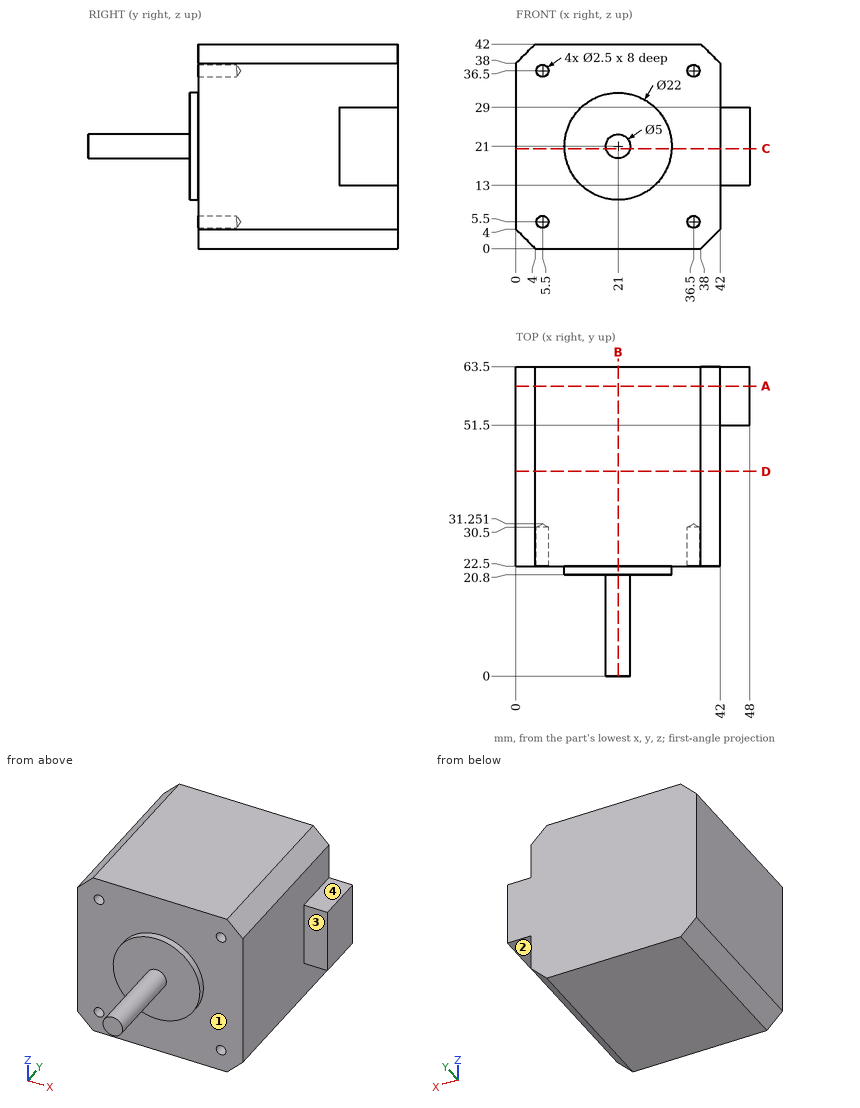
Print and shaded views of the part. All mm, measured from the part's lowest x, y and z. A direction names the side the tool comes from. Coordinates: 2 decimals unless noted, no trailing zeros. Loops run counter-clockwise (first coordinate to the right, second up) from the corner with the lowest first, then second, coordinate; pieces in that order, holes last. Notation, with made-up numbers: (15.25, 44.25) - (35.25, 44.25) arc R23 cw to (35.25, 56.25) - close; hole circle Ø3 at (-5, -13). An arc over 180 degrees is marked (long way). Write item = value, one per line. Start each with the question number.
Item 1: Cut at D-D, the plane y = 42. Give the cut face in (x, z).
Item 2: Cut at B-B, the plane x = 21. Give the cut face in (y, z), and give its area (3 significant figures).
Item 3: 3-axis set-ups, long thin cutter, end or side, ignore diameter. For the marked faces 1, 2, 3 and 4: which of +Z, -Z, +X, -X, +Y, -Y reach the whole face in a straight line?
Item 4: Wall check: L1, parallel to X at y = 25.5, z = 5.5; L2, parallel to X at y = 28, z = 36. Give the ranges that are in metal, low to high. Write a range as from..to.
Item 5: Cut at C-C, the plane z = 20.5. Give the cut face in (x, y).
Item 6: Flat gauge pins, fed straight in: pin 1 Ø5 at (x, y) = (46, 60) entering from +Z; pin 2 Ø1.8 at (x, y) = (45.5, 54.5) entering from -Z; pin 3 Ø1 at (y, z) = (25, 7.5) entering from +X; pin 4 Ø11 at (x, z) = (22.5, 21.5) entering from -Y. Where does each tip first touch, or does it go through?
Item 7: Cut at A-A, the plane y = 59.5. Give the cut face in (x, z).
The answers:
q1.outline = (0, 4) - (4, 0) - (38, 0) - (42, 4) - (42, 38) - (38, 42) - (4, 42) - (0, 38) - close
q2.outline = (0, 18.5) - (20.8, 18.5) - (20.8, 10) - (22.5, 10) - (22.5, 0) - (63.5, 0) - (63.5, 42) - (22.5, 42) - (22.5, 32) - (20.8, 32) - (20.8, 23.5) - (0, 23.5) - close
q2.area = 1,860 mm2
q3.face_1 = -Y
q3.face_2 = -Z, +X, +Y, -Y
q3.face_3 = +Z, -Z, +X, -Y
q3.face_4 = +Z, +X, +Y, -Y
q4.L1 = 0..4.25, 6.75..35.25, 37.75..42
q4.L2 = 0..4.35, 6.65..35.35, 37.65..42
q5.outline = (0, 22.5) - (10.01, 22.5) - (10.01, 20.8) - (18.55, 20.8) - (18.55, 0) - (23.45, 0) - (23.45, 20.8) - (31.99, 20.8) - (31.99, 22.5) - (42, 22.5) - (42, 51.5) - (48, 51.5) - (48, 63.5) - (0, 63.5) - close
q6.pin_1 = 29
q6.pin_2 = 13
q6.pin_3 = 42
q6.pin_4 = 0
q7.outline = (0, 4) - (4, 0) - (38, 0) - (42, 4) - (42, 13) - (48, 13) - (48, 29) - (42, 29) - (42, 38) - (38, 42) - (4, 42) - (0, 38) - close
